Autodesk Fusion 360 part; units mm, degrees
sketch "Sketch1" plane through (0, 0, 0) normal (0, 0, 1) x (1, 0, 0)
  line L0 (-125, 200) -> (125, 200)
  line L1 (125, 200) -> (125, -200)
  line L2 (125, -200) -> (-125, -200)
  line L3 (-125, -200) -> (-125, 200)
  dimension "d1" = 250
  dimension "d2" = 400
extrude "Extrude1" add sketch "Sketch1" along normal blind 200
sketch "Sketch2" plane through (0, 0, 200) normal (0, 0, 1) x (-1, 0, 0)
  line L0 (125, 200) -> (-125, 200)
  line L1 (-125, 200) -> (-125, -200)
  line L2 (-125, -200) -> (125, -200)
  line L3 (125, -200) -> (125, 200)
  line L4 (115, -190) -> (-115, -190)
  line L5 (-115, -190) -> (-115, 190)
  line L6 (-115, 190) -> (115, 190)
  line L7 (115, 190) -> (115, -190)
  dimension "d5" = 230
  dimension "d6" = 380
extrude "Extrude2" cut sketch "Sketch2" against normal blind 180 contours L4 L5 L6 L7
fillet "Fillet1" radius 20 4 edges at (-125, -200, 100) (125, -200, 100) (125, 200, 100) (-125, 200, 100)
fillet "Fillet2" radius 20 4 edges at (115, -190, 110) (-115, -190, 110) (115, 190, 110) (-115, 190, 110)
CAD build for the part. Positions are in the model's coordinates, mm. A direction names the side the tool comes from. Coordinates: 2 decimals unless noted, no trailing zeros. Order: outer loops, then holes, each group sorted by start corner. A loop starts at its lowest first (then second) coordinate and runs counter-clockwise, first axis right, second up.
(1) Pin check, flat tip, straight feed: pin 1 Ø3 at (x, y) = (-63, 6.5) entering from -Z. Stop position of the tip, or through.
Solution:
pin 1: stops at z = 0
(2) Saw through at A-A, the plane x = -32. Write the cut outline in (y, z).
Solution:
outline: (-200, 0) - (200, 0) - (200, 200) - (190, 200) - (190, 20) - (-190, 20) - (-190, 200) - (-200, 200) - close
(3) Drill centre lines: L1, parallel to Y at x = 9, z = 95; L2, parallel to X at y = -130.5, z = 71; L3, parallel to Z at x = 40, y = 140.5. Where is each one in solid material? Low to high.
Solution:
L1: y = -200 to -190, 190 to 200
L2: x = -125 to -115, 115 to 125
L3: z = 0 to 20
(4) Which spindle directions (+Z, -Z, +X, -X, +Y, -Y) get a long thin tool onto all of the face, cutting with end or side? Do faces 5 (the face through (-121, 1, 200)), 6 (the face through (-1, 190, 111)). Say none if no direction does.
Solution:
face 5: +Z, +X, -X, +Y, -Y
face 6: +Z
(5) Saw through at C-C, the plane y = -106.5. Write the cut outline in (x, z), and give its area (3 significant figures).
Solution:
outline: (-125, 0) - (125, 0) - (125, 200) - (115, 200) - (115, 20) - (-115, 20) - (-115, 200) - (-125, 200) - close
area: 8,600 mm2
(6) Mould opens along Y. For faces 1 (the face through (-2, 3, 0)), 2 (the face through (1, -200, 99)), 3 (the face through (-1, 200, 99)), 4 (the face through (109.297, -183.986, 108.74)) say: released by +Y, released by -Y, zero draft, split by the parting line, or undercut.
Solution:
face 1: zero draft
face 2: released by -Y
face 3: released by +Y
face 4: undercut
(7) Saw through at B-B, the plane z = 37. Write the cut outline in (x, y).
Solution:
outline: (-125, -180) arc R20 ccw to (-105, -200) - (105, -200) arc R20 ccw to (125, -180) - (125, 180) arc R20 ccw to (105, 200) - (-105, 200) arc R20 ccw to (-125, 180) - close; hole (-115, -170) arc R20 ccw to (-95, -190) - (95, -190) arc R20 ccw to (115, -170) - (115, 170) arc R20 ccw to (95, 190) - (-95, 190) arc R20 ccw to (-115, 170) - close
